Can you work these out from the model? Positions are in its coordinate system, mm. A direction names the side the tool comes from. Round coordinates to 2 decimals unless told otherwise and drop trailing zeros. Order: outer loops, then holes, each group sorted by start corner. A loop starts at its lowest first (then second) coordinate and runs counter-clockwise, first axis right, second up. Notation, with made-up numbers: (26, 86) -> (63, 86) arc R20 ccw to (63, 125) -> close; hole circle Ø5 at (-21.75, -31). An arc over 180 degrees is marked (long way). One line per item, written item: value.
```python
from build123d import *

# Parameters (mm, degrees)
IZIM2_W                       = 100
IZIM2_H                       = 90
Y_KSEKLIK_EKSTR_ZYON1_DEPTH   = 30
KES_EKSTR_ZYON11_DEPTH        = 22
KES_EKSTR_ZYON12_DEPTH        = 22
IZIM7_W                       = 12.5
IZIM7_H                       = 16.5
KES_EKSTR_ZYON13_DEPTH        = 70
IZIM8_W                       = 6
IZIM8_H                       = 30
KES_EKSTR_ZYON14_DEPTH        = 100
IZIM9_W                       = 22
IZIM9_H                       = 6
KES_EKSTR_ZYON15_DEPTH        = 100
IZIM10_W                      = 12
IZIM10_H                      = 10
KES_EKSTR_ZYON16_DEPTH        = 100
IZIM11_W                      = 12
IZIM11_H                      = 10
KES_EKSTR_ZYON17_DEPTH        = 45
Y_KSEKLIK_EKSTR_ZYON2_DEPTH   = 45
Y_KSEKLIK_EKSTR_ZYON2_2_DEPTH = 45
IZIM13_W                      = 9.7
IZIM13_H                      = 15.2
KES_EKSTR_ZYON18_DEPTH        = 45
IZIM14_W                      = 9.7
IZIM14_H                      = 15.2
KES_EKSTR_ZYON19_DEPTH        = 45
IZIM15_W                      = 64.648209686
IZIM15_H                      = 50.718484946
KES_EKSTR_ZYON20_DEPTH        = 45
KES_EKSTR_ZYON21_DEPTH        = 100
IZIM17_R                      = 1.1
KES_EKSTR_ZYON24_DEPTH        = 100
KES_EKSTR_ZYON25_DEPTH        = 100


with BuildPart() as part:
    # Çizim2 → Yükseklik-Ekstrüzyon1 (new body)
    with BuildSketch(Plane(origin=(0, 0, 0), x_dir=(1, 0, 0), z_dir=(0, 1, 0))):
        with Locations((-5.3298184, 8.1959709)):
            Rectangle(IZIM2_W, IZIM2_H)
    extrude(amount=Y_KSEKLIK_EKSTR_ZYON1_DEPTH)

    # Çizim5 → Kes-Ekstrüzyon11 (cut)
    with BuildSketch(Plane(origin=(44.6701816, 0, 0), x_dir=(0, 0, -1), z_dir=(1, 0, 0))):
        with BuildLine():
            Line((36.1959709, 29), (53.1959709, 29))
            Line((53.1959709, 29), (53.1959709, 0))
            Line((53.1959709, 0), (24.154376321, 0))
            ThreePointArc((24.154376321, 0), (20.495652432, 18.519202405), (36.1959709, 29))
        make_face()
    extrude(amount=-KES_EKSTR_ZYON11_DEPTH, mode=Mode.SUBTRACT)

    # Çizim6 → Kes-Ekstrüzyon12 (cut)
    with BuildSketch(Plane.ZY.offset(55.3298184)):
        with BuildLine():
            Line((-36.1959709, 29), (-53.1959709, 29))
            Line((-53.1959709, 29), (-53.1959709, 0))
            Line((-53.1959709, 0), (-24.154376321, 0))
            ThreePointArc((-24.154376321, 0), (-20.495652432, 18.519202405), (-36.1959709, 29))
        make_face()
    extrude(amount=-KES_EKSTR_ZYON12_DEPTH, mode=Mode.SUBTRACT)

    # Çizim7 → Kes-Ekstrüzyon13 (cut)
    with BuildSketch(Plane(origin=(22.6701816, 0, 0), x_dir=(0, 0, -1), z_dir=(1, 0, 0))):
        with Locations((36.1959709, 12)):
            Rectangle(IZIM7_W, IZIM7_H)
    extrude(amount=-KES_EKSTR_ZYON13_DEPTH, mode=Mode.SUBTRACT)

    # Çizim8 → Kes-Ekstrüzyon14 (cut)
    with BuildSketch(Plane(origin=(22.6701816, 0, 0), x_dir=(0, 0, -1), z_dir=(1, 0, 0))):
        with Locations((50.1959709, 15)):
            Rectangle(IZIM8_W, IZIM8_H)
    extrude(amount=-KES_EKSTR_ZYON14_DEPTH, mode=Mode.SUBTRACT)

    # Çizim9 → Kes-Ekstrüzyon15 (cut)
    with BuildSketch(Plane(origin=(0, 30, 0), x_dir=(1, 0, 0), z_dir=(0, 1, 0))):
        with Locations((33.6701816, 50.1959709)):
            Rectangle(IZIM9_W, IZIM9_H)
    extrude(amount=-KES_EKSTR_ZYON15_DEPTH, mode=Mode.SUBTRACT)

    # Çizim10 → Kes-Ekstrüzyon16 (cut)
    with BuildSketch(Plane(origin=(44.6701816, 0, 0), x_dir=(0, 0, -1), z_dir=(1, 0, 0))):
        with Locations((4.1959709, 10)):
            Rectangle(IZIM10_W, IZIM10_H)
    extrude(amount=-KES_EKSTR_ZYON16_DEPTH, mode=Mode.SUBTRACT)

    # Çizim11 → Kes-Ekstrüzyon17 (cut)
    with BuildSketch(Plane.XY.offset(36.8040291)):
        with Locations((-5.3298184, 10)):
            Rectangle(IZIM11_W, IZIM11_H)
    extrude(amount=-KES_EKSTR_ZYON17_DEPTH, mode=Mode.SUBTRACT)

    # Çizim13 → Kes-Ekstrüzyon18 (cut)
    with BuildSketch(Plane(origin=(12.73710535, 0, 12.73710535), x_dir=(0.707106781, 0, -0.707106781), z_dir=(0.707106781, 0, 0.707106781))):
        with Locations((-38.885769972, 12.6)):
            Rectangle(IZIM13_W, IZIM13_H)
    extrude(amount=-KES_EKSTR_ZYON18_DEPTH, mode=Mode.SUBTRACT)

    # Çizim14 → Kes-Ekstrüzyon19 (cut)
    with BuildSketch(Plane(origin=(-18.06692375, 0, 18.06692375), x_dir=(0.707106781, 0, 0.707106781), z_dir=(-0.707106781, 0, 0.707106781))):
        with Locations((31.348268505, 12.6)):
            Rectangle(IZIM14_W, IZIM14_H)
    extrude(amount=-KES_EKSTR_ZYON19_DEPTH, mode=Mode.SUBTRACT)

    # Çizim16 → Kes-Ekstrüzyon21 (cut)
    with BuildSketch(Plane(origin=(44.6701816, 0, 0), x_dir=(0, 0, -1), z_dir=(1, 0, 0))):
        Polygon((-36.8040291, 0), (-26.8040291, 3), (-18.8040291, 15), (1.1959709, 30), (-36.8040291, 30), align=None)
    extrude(amount=-KES_EKSTR_ZYON21_DEPTH, mode=Mode.SUBTRACT)

    # Çizim17 → Kes-Ekstrüzyon24 (cut)
    with BuildSketch(Plane(origin=(0, 30, 0), x_dir=(1, 0, 0), z_dir=(0, 1, 0))):
        with Locations((-28.3298184, 42.1959709)):
            Circle(IZIM17_R)
        with Locations((-45.3298184, 16.1959709)):
            Circle(IZIM17_R)
        with Locations((34.6701816, 16.1959709)):
            Circle(IZIM17_R)
        with Locations((17.6701816, 42.1959709)):
            Circle(IZIM17_R)
    extrude(amount=-KES_EKSTR_ZYON24_DEPTH, mode=Mode.SUBTRACT)

    # Çizim19 → Kes-Ekstrüzyon25 (cut)
    with BuildSketch(Plane(origin=(0, 0, -47.1959709), x_dir=(-1, 0, 0), z_dir=(0, 0, -1))):
        Polygon((-44.6701816, 0), (-37.1701816, 30), (-44.6701816, 30), align=None)
        Polygon((55.3298184, 0), (55.3298184, 30), (47.8298184, 30), align=None)
    extrude(amount=-KES_EKSTR_ZYON25_DEPTH, mode=Mode.SUBTRACT)


with BuildPart() as body_2:
    # Çizim12 → Yükseklik-Ekstrüzyon2 (new body)
    with BuildSketch(Plane(origin=(0, 30, 0), x_dir=(1, 0, 0), z_dir=(0, 1, 0))):
        Polygon((-11.3298184, -36.8040291), (-17.233785956, -42.707996656), (-17.233785956, -36.8040291), align=None)
    extrude(amount=Y_KSEKLIK_EKSTR_ZYON2_DEPTH)


with BuildPart() as body_3:
    # Çizim12 → Y_kseklik-Ekstr_zyon2 2 (new body)
    with BuildSketch(Plane(origin=(0, 30, 0), x_dir=(1, 0, 0), z_dir=(0, 1, 0))):
        Polygon((0.6701816, -36.8040291), (4.718486826, -40.852334326), (4.718486826, -36.8040291), align=None)
    extrude(amount=Y_KSEKLIK_EKSTR_ZYON2_2_DEPTH)


with BuildPart() as kes_ekstr_zyon20_tool:
    # Çizim15 → Kes-Ekstrüzyon20 (new body)
    with BuildSketch(Plane(origin=(0, 30, 0), x_dir=(1, 0, 0), z_dir=(0, 1, 0))):
        with Locations((5.316439318, -44.683310577)):
            Rectangle(IZIM15_W, IZIM15_H)
    extrude(amount=KES_EKSTR_ZYON20_DEPTH)


with BuildPart() as body_2_1:
    add(body_2.part)

    # Kes-Ekstrüzyon20: cut by kes_ekstr_zyon20_tool
    add(kes_ekstr_zyon20_tool.part, mode=Mode.SUBTRACT)


with BuildPart() as body_3_1:
    add(body_3.part)

    # Kes-Ekstrüzyon20: cut by kes_ekstr_zyon20_tool
    add(kes_ekstr_zyon20_tool.part, mode=Mode.SUBTRACT)


solid = part.part
```
Q1. I want a section at B-B on x = -13. List the corners of the cut face in (y, z) for me.
Answers below:
outline: (0, -47.2) -> (30, -47.2) -> (30, -1.2) -> (15, 18.8) -> (3, 26.8) -> (0, 36.8) -> close; hole (3.75, -42.45) -> (20.25, -42.45) -> (20.25, -29.95) -> (3.75, -29.95) -> close; hole (5, -10.2) -> (15, -10.2) -> (15, 1.8) -> (5, 1.8) -> close
Q2. I want a section at A-A on y = 18.25. List the corners of the cut face in (x, z) for me.
Answers below:
outline: (-50.77, -20.39) -> (-33.33, -20.39) -> (-33.33, -29.95) -> (22.67, -29.95) -> (22.67, -20.39) -> (40.11, -20.39) -> (40.11, 14.47) -> (36.72, 14.47) -> (39.35, 11.84) -> (32.49, 4.98) -> (23, 14.47) -> (-33.66, 14.47) -> (-43.15, 4.98) -> (-50.01, 11.84) -> (-47.38, 14.47) -> (-50.77, 14.47) -> close; (-33.33, -47.2) -> (22.67, -47.2) -> (22.67, -42.45) -> (18.74, -42.45) arc R1.1 cw to (16.6, -42.45) -> (-27.26, -42.45) arc R1.1 cw to (-29.4, -42.45) -> (-33.33, -42.45) -> close; hole circle Ø2.2 at (-45.33, -16.2); hole circle Ø2.2 at (34.67, -16.2)
Q3. We'd pull the mould along Y, two halves only. Please class faces 4 (the face through (28, 5, 16)), 5 (the face through (30, 29, -42)), 6 (the face through (-4.64, 3.583, 26.416)), 7 (the face through (-28.473, 15.21, -43.287)): released by +Y, released by -Y, zero draft, split by the parting line, or undercut.
Answers below:
face 4: undercut
face 5: released by -Y
face 6: released by +Y
face 7: zero draft
Q4. I want a section at D-D on z = -37.5. List the corners of the cut face in (x, y) for me.
Answers below:
outline: (-48.08, 29) -> (-33.33, 29) -> (-33.33, 20.25) -> (22.67, 20.25) -> (22.67, 29) -> (37.42, 29) -> (37.17, 30) -> (-47.83, 30) -> close; (-33.33, 0) -> (22.67, 0) -> (22.67, 3.75) -> (-33.33, 3.75) -> close
Q5. On a 3-axis mill with a long thin cutter (end or side, diameter ignored), from which of +Z, -Z, +X, -X, +Y, -Y can I reach the whole of each face in a straight line? I mean faces 1 (the face through (-5, 15, -2)), 2 (the face through (22, 10, 1.804)), 3 (the face through (31.38, 18.26, -20.39)). Say none if no direction works.
Answers below:
face 1: none
face 2: +X, -X
face 3: -Z, +X
Q6. I want a section at C-C on y = 8.75. Give the number of separate pieces and of enclosed holes in the cut face, plus the area to 3 significant figures.
Answers below:
separate pieces: 4
enclosed holes: 2
area: 3,100 mm^2
Q7. Will these pins go through, and if not, where does the flat tip stop? pin 1 Ø5 at (y, z) = (8.5, 15) entering from +X; pin 2 Ø5.5 at (x, z) = (29.5, -39.5) entering from -Y; pin 3 Ø4 at (y, z) = (10, 1.5) entering from +X.
Answers below:
pin 1: x = 43.17
pin 2: y = 29
pin 3: x = 42.66
Q8. Please list where these lines run through material, in increasing order: line 1 along Y through (x, z) = (-11, -41); line 2 along Z through (x, y) = (-41, 8.5); line 3 along Z through (x, y) = (21, 14.5).
Answers below:
line 1: 0 to 3.75, 20.25 to 30
line 2: -19.56 to -10.2, 1.8 to 7.13, 20.85 to 23.14
line 3: -47.2 to -42.45, -29.95 to -10.2, 1.8 to 16.47
